Check sheet for the modelled part. Datum: model origin and axes. Units: mm. Coordinates: 2 decimals unless noted, no trailing zeros. Write each loop counter-clockwise with the first axis right and the second up, starting at its lowest first coordinate (ties: lowest second). Pieces come first, ordered by that corner, then holes. Notation, with made-up numbers: (77, -6.75) - (91, -6.75) arc R17 cw to (91, 10.25) - close; hole circle Ø6 at (52.25, -28.5). An arc over 180 degrees is marked (long way). Use one line per item in the form item = value. Start each with the question number.
1. Cross-section at D-D on y = 1.2. Record the boundary of the cut face in (x, z).
2. Go/stop test with a flat-tipped pin: pin 1 Ø2 at (x, z) = (1.5, 9) entering from +Y (3 decimals). Record where the tip stops, or that it passes through.
3. Cross-section at A-A on y = 0.4. Record the boundary of the cut face in (x, z), then the cut area to 3 significant figures.
4. Cross-section at B-B on x = 0. Record the boundary of the cut face in (y, z).
5. Scan lines: line 1 along Y through (x, z) = (0, 5.25); line 2 along Y through (x, z) = (0.55, 9.5); line 3 along X through (y, z) = (1.15, 0.75). Record each from-to range of solid material in increasing order.
```python
from build123d import *

# Parameters (mm, degrees)
F1_DEPTH = 10
F2_R     = 0.39999


# Not quite as in the source:
# - a fillet or chamfer is up to 0.001 mm smaller than in the source, because OpenCascade refuses the exact size


with BuildPart() as f1:
    # F0 (on Top) → F1 (new body)
    with BuildSketch(Plane.XY):
        with BuildLine():
            ThreePointArc((-1.1635984277, -0.9465932067), (-0.502295908, 1.4133997385), (1.5, 0))
            ThreePointArc((1.5, 0), (1.1417008858, -0.9728921252), (0.2379745502, -1.4810024016))
            Line((0.2379745502, -1.4810024016), (0.3648943103, -2.2708703491))
            ThreePointArc((0.3648943103, -2.2708703491), (1.7506080249, -1.4917679254), (2.3, 0))
            ThreePointArc((2.3, 0), (-0.7701870589, 2.1672129324), (-1.7841842559, -1.4514429169))
            Line((-1.7841842559, -1.4514429169), (-1.1635984277, -0.9465932067))
        make_face()
    extrude(amount=F1_DEPTH)

    # F2 (radius 0.4 in the source; OpenCascade refuses exactly that, so slightly less here)
    f2_edges = [f1.edges().sort_by_distance(p)[0] for p in [
        (-1.784184, -1.451443, 5),
        (-1.163598, -0.946593, 5),
        (-1.473891, -1.199018, 0),
        (-1.473891, -1.199018, 10),
        (0.237975, -1.481002, 5),
        (0.364894, -2.27087, 5),
        (0.301434, -1.875936, 0),
        (0.301434, -1.875936, 10),
    ]]
    fillet(f2_edges, radius=F2_R)


solid = f1.part
```
Final values:
q1.outline = (-1.96, 0) - (-0.9, 0) - (-0.9, 10) - (-1.96, 10) - close; (0.9, 0) - (1.96, 0) - (1.96, 10) - (0.9, 10) - close
q2.pin_1 = 2.245
q3.outline = (-2.26, 0) - (-1.45, 0) - (-1.45, 10) - (-2.26, 10) - close; (1.45, 0) - (2.26, 0) - (2.26, 10) - (1.45, 10) - close
q3.area = 16.4 mm²
q4.outline = (1.5, 0) - (2.3, 0) - (2.3, 10) - (1.5, 10) - close
q5.line_1 = 1.5 to 2.3
q5.line_2 = -2.15 to -1.4, 1.4 to 2.23
q5.line_3 = -1.99 to -0.96, 0.96 to 1.99
